from build123d import *

# Parameters (mm, degrees)
SKETCH_1_R               = 16
EXTRUDE_1_DEPTH          = 3
SKETCH_2_R               = 8
EXTRUDE_2_DEPTH          = 10
SKETCH_3_R               = 5
CUT_EXTRUDE_1_DEPTH      = 27.095976701
SKETCH_4_R               = 2
CUT_EXTRUDE_2_DEPTH      = 7
CUT_EXTRUDE_3_DEPTH      = 27.095976701
CUT_EXTRUDE_3_DEPTH_BACK = 27.095976701
SKETCH_5_R               = 2
FILLET_1_R               = 0.5
FILLET_2_R               = 0.5


with BuildPart() as part:
    # 草图1 → 凸台-拉伸1 (new body)
    with BuildSketch(Plane(origin=(0, 0, 0), x_dir=(1, 0, 0), z_dir=(0, 1, 0))):
        with Locations(Location((0, 0, 0), (0, 0, 270))):
            Circle(SKETCH_1_R)
    extrude(amount=EXTRUDE_1_DEPTH)

    # 草图2 → 凸台-拉伸2 (add)
    with BuildSketch(Plane(origin=(0, 3, 0), x_dir=(1, 0, 0), z_dir=(0, 1, 0))):
        with Locations(Location((0, 0, 0), (0, 0, 270))):
            Circle(SKETCH_2_R)
    extrude(amount=EXTRUDE_2_DEPTH)

    # 草图3 → 切除-拉伸1 (cut, through all)
    with BuildSketch(Plane(origin=(0, 13, 0), x_dir=(1, 0, 0), z_dir=(0, 1, 0))):
        with Locations(Location((0, 0, 0), (0, 0, 270))):
            Circle(SKETCH_3_R)
    extrude(amount=-CUT_EXTRUDE_1_DEPTH, mode=Mode.SUBTRACT)

    # 草图4 → 切除-拉伸2 (cut)
    with BuildSketch(Plane(origin=(0, 3, 0), x_dir=(1, 0, 0), z_dir=(0, 1, 0))):
        with Locations(Location((0, 13, 0), (0, 0, 270))):
            Circle(SKETCH_4_R)
        with Locations(Location((-13, 0, 0), (0, 0, 270))):
            Circle(SKETCH_4_R)
        with Locations(Location((0, -13, 0), (0, 0, 270))):
            Circle(SKETCH_4_R)
        with Locations(Location((13, 0, 0), (0, 0, 270))):
            Circle(SKETCH_4_R)
    extrude(amount=-CUT_EXTRUDE_2_DEPTH, mode=Mode.SUBTRACT)

    # 草图5 → 切除-拉伸3 (cut, two sides: drawn at the far end of the back side and taken through both)
    with BuildSketch(Plane(origin=(0, 0, 0), x_dir=(0, 0, -1), z_dir=(1, 0, 0)).offset(-CUT_EXTRUDE_3_DEPTH_BACK)):
        with Locations((0, 7.5)):
            Circle(SKETCH_5_R)
    extrude(amount=CUT_EXTRUDE_3_DEPTH + CUT_EXTRUDE_3_DEPTH_BACK, mode=Mode.SUBTRACT)

    # 圆角1
    fillet_1_edges = [part.edges().sort_by_distance(p)[0] for p in [
        (0, 3, -16),
    ]]
    fillet(fillet_1_edges, radius=FILLET_1_R)

    # 圆角2
    fillet_2_edges = [part.edges().sort_by_distance(p)[0] for p in [
        (0, 13, -8),
    ]]
    fillet(fillet_2_edges, radius=FILLET_2_R)


solid = part.part
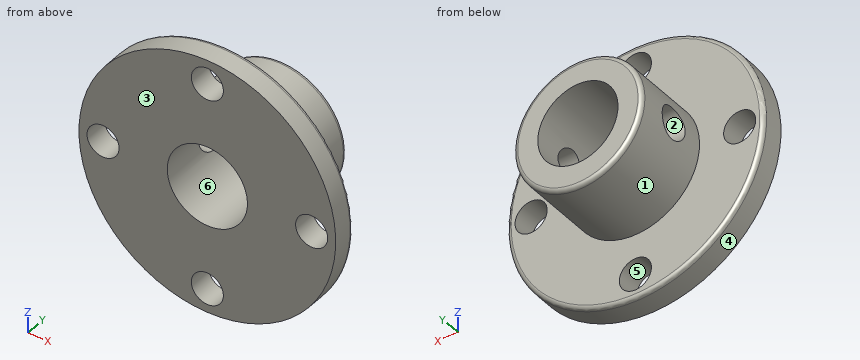
Build history of the part. All positions in model axes, mm. Face numbers are marked on the shaded views. A direction names the side the tool comes from. Round coordinates to 2 decimals unless told otherwise and drop trailing zeros. Write each loop counter-clockwise with the first axis right and the second up, starting at its lowest first coordinate (ties: lowest second). Pieces come first, ordered by that corner, then holes. Notation, with made-up numbers: M -13,6 L 5,6 A20 ccw 5,37 Z; hole C -16,74.25 d9. An arc over 180 degrees is marked long. Answer as a JSON object with one key per item and string values. Group by question number.
(1) Mould opens along Z. For the marked faces 3, 4, 5 and 6 say: pulls with the +Z half, pulls with the -Z half, needs draft (parallel to the pull), parting line crosses it, or undercut.
(2) Drill centre lines: L1, parallel to X at y = 2.35, z = 0; L2, parallel to X at y = 2.1, z = 13; L3, parallel to X at y = 0.5, z = -4.5. Where is each one in solid material? Low to high.
(3) Flat gauge pins, fed straight in: pin 1 (11.5 mm diameter, centred on x = 0, z = 0, fed in from -Y); pin 2 (3 mm diameter, centred on y = 4, z = 3, fed in from -X); pin 3 (5 mm diameter, centred on y = 6, z = 7, fed in from -X); pin 4 (5 mm diameter, centred on y = 7.5, z = 0, fed in from -X). Where does each tip first touch, or does it go through?
(4) Which spindle directions (+Z, -Z, +X, -X, +Y, -Y) get a long thin tool onto all of the face, cutting with end or side? Do the marked faces 1 and 2. Say none if no direction does.
(5) Cut at A-A (x = -1). Give the number of separate pieces and of enclosed holes in the cut face, and give its area (3 significant figures).
(6) Cut at B-B (y = 12). Give the cut face in (x, z).
Responses:
{
 "1": {"face 3": "needs draft", "face 4": "parting line crosses it", "face 5": "undercut", "face 6": "undercut"},
 "2": {"L1": "x = -16 to -15, -11 to -5, 5 to 11, 15 to 16", "L2": "x = -9.33 to -2, 2 to 9.33", "L3": "x = -15.35 to -2.18, 2.18 to 15.35"},
 "3": {"pin 1": "stops at y = 0", "pin 2": "stops at x = -15.8", "pin 3": "stops at x = -6.61", "pin 4": "stops at x = -8"},
 "4": {"face 1": "+Y", "face 2": "+X, -X"},
 "5": {"separate pieces": "4", "enclosed holes": "0", "area": "106 mm2"},
 "6": {"outline": "C 0,0 d16; hole C 0,0 d10"}
}
